from build123d import *

# Parameters (mm, degrees)
SKETCH_1_R          = 30
SKETCH_1_R_2        = 2
EXTRUDE_1_DEPTH     = 5.2
SKETCH_2_R          = 14
EXTRUDE_2_DEPTH     = 0.4
SKETCH_3_R          = 10
EXTRUDE_3_DEPTH     = 16
SKETCH_4_R          = 2.5
CUT_EXTRUDE_1_DEPTH = 12
CHAMFER_1_SIZE      = 1.7


with BuildPart() as part:
    # 草图1 → 凸台-拉伸1 (new body)
    with BuildSketch(Plane.XY):
        with Locations((0, 0.477974548)):
            Circle(SKETCH_1_R)
        with Locations((0, 22)):
            Circle(SKETCH_1_R_2, mode=Mode.SUBTRACT)
        with Locations((-12.374368671, 12.374368671)):
            Circle(SKETCH_1_R_2, mode=Mode.SUBTRACT)
        with Locations((22, 0)):
            Circle(SKETCH_1_R_2, mode=Mode.SUBTRACT)
        with Locations((12.374368671, 12.374368671)):
            Circle(SKETCH_1_R_2, mode=Mode.SUBTRACT)
        with Locations((0, -22)):
            Circle(SKETCH_1_R_2, mode=Mode.SUBTRACT)
        with Locations((12.374368671, -12.374368671)):
            Circle(SKETCH_1_R_2, mode=Mode.SUBTRACT)
        with Locations((-22, 0)):
            Circle(SKETCH_1_R_2, mode=Mode.SUBTRACT)
        with Locations((-12.374368671, -12.374368671)):
            Circle(SKETCH_1_R_2, mode=Mode.SUBTRACT)
    extrude(amount=EXTRUDE_1_DEPTH)

    # 草图2 → 凸台-拉伸2 (add)
    with BuildSketch(Plane.XY.offset(5.2)):
        Circle(SKETCH_2_R)
    extrude(amount=EXTRUDE_2_DEPTH)

    # 草图3 → 凸台-拉伸3 (add)
    with BuildSketch(Plane.XY.offset(5.6)):
        Circle(SKETCH_3_R)
    extrude(amount=EXTRUDE_3_DEPTH)

    # 草图4 → 切除-拉伸1 (cut)
    with BuildSketch(Plane.XY.offset(21.6)):
        Circle(SKETCH_4_R)
    extrude(amount=-CUT_EXTRUDE_1_DEPTH, mode=Mode.SUBTRACT)

    # 倒角1
    # the kernel refuses this chamfer: 1.7 mm, written as the material it takes off along each edge
    with BuildSketch(Plane(origin=(22, 0, 5.2), x_dir=(1, 0, 0), z_dir=(0, -1, 0))) as chamfer_1_piece_1:
        Polygon((2 + CHAMFER_1_SIZE, 0), (2, -CHAMFER_1_SIZE), (2, 0), align=None)
    revolve(axis=Axis((22, 0, 5.2), (0, 0, 1)), mode=Mode.SUBTRACT)
    with BuildSketch(Plane(origin=(12.374368671, 12.374368671, 5.2), x_dir=(1, 0, 0), z_dir=(0, -1, 0))) as chamfer_1_piece_2_section:
        Polygon((2 + CHAMFER_1_SIZE, 0), (2, -CHAMFER_1_SIZE), (2, 0), align=None)
    chamfer_1_piece_2 = revolve(axis=Axis((12.374368671, 12.374368671, 5.2), (0, 0, 1)), mode=Mode.PRIVATE)
    chamfer_1_piece_2 = chamfer_1_piece_2 - Plane(origin=(0, 0, 4.370822152), x_dir=(1, 0, 0), z_dir=(0, 0, -1)) * Cylinder(14, 15, mode=Mode.PRIVATE)
    add(chamfer_1_piece_2, mode=Mode.SUBTRACT)
    with BuildSketch(Plane(origin=(0, -22, 5.2), x_dir=(1, 0, 0), z_dir=(0, -1, 0))) as chamfer_1_piece_3:
        Polygon((2 + CHAMFER_1_SIZE, 0), (2, -CHAMFER_1_SIZE), (2, 0), align=None)
    revolve(axis=Axis((0, -22, 5.2), (0, 0, 1)), mode=Mode.SUBTRACT)
    with BuildSketch(Plane(origin=(12.374368671, -12.374368671, 5.2), x_dir=(1, 0, 0), z_dir=(0, -1, 0))) as chamfer_1_piece_4_section:
        Polygon((2 + CHAMFER_1_SIZE, 0), (2, -CHAMFER_1_SIZE), (2, 0), align=None)
    chamfer_1_piece_4 = revolve(axis=Axis((12.374368671, -12.374368671, 5.2), (0, 0, 1)), mode=Mode.PRIVATE)
    chamfer_1_piece_4 = chamfer_1_piece_4 - Plane(origin=(0, 0, 4.370822149), x_dir=(1, 0, 0), z_dir=(0, 0, -1)) * Cylinder(14, 15, mode=Mode.PRIVATE)
    add(chamfer_1_piece_4, mode=Mode.SUBTRACT)
    with BuildSketch(Plane(origin=(-22, 0, 5.2), x_dir=(1, 0, 0), z_dir=(0, -1, 0))) as chamfer_1_piece_5:
        Polygon((2 + CHAMFER_1_SIZE, 0), (2, -CHAMFER_1_SIZE), (2, 0), align=None)
    revolve(axis=Axis((-22, 0, 5.2), (0, 0, 1)), mode=Mode.SUBTRACT)
    with BuildSketch(Plane(origin=(-12.374368671, -12.374368671, 5.2), x_dir=(1, 0, 0), z_dir=(0, -1, 0))) as chamfer_1_piece_6_section:
        Polygon((2 + CHAMFER_1_SIZE, 0), (2, -CHAMFER_1_SIZE), (2, 0), align=None)
    chamfer_1_piece_6 = revolve(axis=Axis((-12.374368671, -12.374368671, 5.2), (0, 0, 1)), mode=Mode.PRIVATE)
    chamfer_1_piece_6 = chamfer_1_piece_6 - Plane(origin=(0, 0, 4.370822148), x_dir=(1, 0, 0), z_dir=(0, 0, -1)) * Cylinder(14, 15, mode=Mode.PRIVATE)
    add(chamfer_1_piece_6, mode=Mode.SUBTRACT)
    with BuildSketch(Plane(origin=(0, 22, 0), x_dir=(1, 0, 0), z_dir=(0, -1, 0))) as chamfer_1_piece_7:
        Polygon((2 + CHAMFER_1_SIZE, 0), (2, CHAMFER_1_SIZE), (2, 0), align=None)
    revolve(axis=Axis((0, 22, 0), (0, 0, 1)), mode=Mode.SUBTRACT)
    with BuildSketch(Plane(origin=(0, 22, 5.2), x_dir=(1, 0, 0), z_dir=(0, -1, 0))) as chamfer_1_piece_8:
        Polygon((2 + CHAMFER_1_SIZE, 0), (2, -CHAMFER_1_SIZE), (2, 0), align=None)
    revolve(axis=Axis((0, 22, 5.2), (0, 0, 1)), mode=Mode.SUBTRACT)
    with BuildSketch(Plane(origin=(-12.374368671, 12.374368671, 5.2), x_dir=(1, 0, 0), z_dir=(0, -1, 0))) as chamfer_1_piece_9_section:
        Polygon((2 + CHAMFER_1_SIZE, 0), (2, -CHAMFER_1_SIZE), (2, 0), align=None)
    chamfer_1_piece_9 = revolve(axis=Axis((-12.374368671, 12.374368671, 5.2), (0, 0, 1)), mode=Mode.PRIVATE)
    chamfer_1_piece_9 = chamfer_1_piece_9 - Plane(origin=(0, 0, 4.370822151), x_dir=(1, 0, 0), z_dir=(0, 0, -1)) * Cylinder(14, 15, mode=Mode.PRIVATE)
    add(chamfer_1_piece_9, mode=Mode.SUBTRACT)


solid = part.part
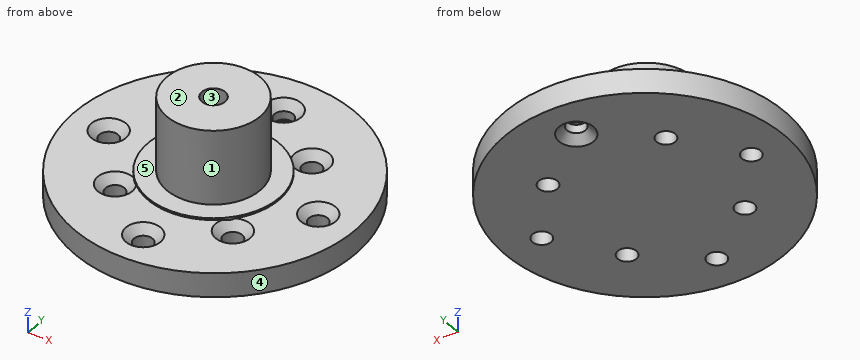
Build history of the part. All positions in model axes, mm. Face numbers are marked on the shaded views. A direction names the side the tool comes from. Coordinates: 2 decimals unless noted, no trailing zeros. Order: outer loops, then holes, each group sorted by start corner. A loop starts at its lowest first (then second) coordinate and runs counter-clockwise, first axis right, second up. Notation, with made-up numbers: M -6.5,71.25 L 33.5,71.25 A19 cw 33.5,103.25 Z; hole C 8.5,73.5 d8. An arc over 180 degrees is marked long. One line per question, with ' | ' between items. Start each with the question number.
Q1. Saw through at D-D (z = 7). List the corners of the cut face in (x, y), then the cut area to 3 significant figures.
Q2. Saw through at B-B (x = -22). List the corners of the cut face in (y, z).
Q3. Saw through at A-A (x = 0). Count the separate pieces of the cut face and the enclosed holes in it, then the cut area to 3 significant figures.
Q4. Two-plate mould, pull along X, no slides. Class the marked faces 1, 2 and 3: +X half, -X half, draft (parallel to the pull), parting line (faces both ways), or undercut.
Q5. Flat gauge pins, fed straight in: pin 1 Ø5 at (y, z) = (-7, 15) entering from +X; pin 2 Ø10 at (y, z) = (5, 8.5) entering from -X; pin 3 Ø5 at (x, y) = (-22, 0) entering from +Z. Where does each tip first touch, or does it go through?
Q6. Probe L1, parallel to Y at x = 0, z = 2.1; L2, parallel to Z at x = -16, y = -0.5; L3, parallel to X at y = -2, z = 20.5. List the from-to ranges inside material, lowest first. Write a range as from..to.
Q7. Saw through at C-C (x = -7). List the corners of the cut face in (y, z).
Q8. 3-axis set-ups, long thin cutter, end or side, ignore diameter. For the marked faces 4 and 5: which of +Z, -Z, +X, -X, +Y, -Y reach the whole face in a straight line?
Check values:
1) outline: C 0,0 d20 | area: 314 mm2
2) outline: M -19.92,0 L -2,0 L -2,3.5 L -3.7,5.2 L -19.92,5.2 Z; M 2,0 L 20.87,0 L 20.87,5.2 L 3.7,5.2 L 2,3.5 Z
3) separate pieces: 3 | enclosed holes: 0 | area: 533 mm2
4) face 1: parting line | face 2: draft | face 3: undercut
5) pin 1: stops at x = 8.93 | pin 2: stops at x = -29.99 | pin 3: stops at z = 4
6) L1: y = -29.52..-24, -20..20, 24..30.48 | L2: z = 0..5.2 | L3: x = -9.8..-1.5, 1.5..9.8
7) outline: M -28.69,0 L 29.65,0 L 29.65,5.2 L 12.12,5.2 L 12.12,5.6 L 7.14,5.6 L 7.14,21.6 L -7.14,21.6 L -7.14,5.6 L -12.12,5.6 L -12.12,5.2 L -28.69,5.2 Z
8) face 4: +Z, -Z | face 5: +Z
